Source: CAD feature listing. Evaluate the final solid. Frame: model axes, mm. A direction names the side the tool comes from. Coordinates: 2 decimals unless noted, no trailing zeros. Loops run counter-clockwise (first coordinate to the right, second up) from the corner with the lowest first, then second, coordinate; pieces in that order, holes last.
Solid Edge part; units mm, degrees
sketch "Sketch1" plane through (0, 0, 0) normal (0, 0, 1) x (1, 0, 0)
  line L0 (-500, -500) -> (500, -500)
  line L1 (500, -500) -> (500, 500)
  line L2 (500, 500) -> (-500, 500)
  line L3 (-500, 500) -> (-500, -500)
extrude "Protrusion1" add sketch "Sketch1" along normal blind 18
sketch "Sketch2" plane through (0, 0, 0) normal (0, 0, -1) x (1, 0, 0)
  circle A0 centre (0, 0) radius 450
extrude "Kihúzás_2" add sketch "Sketch2" along normal blind 18
sketch "Sketch3" plane through (0, 0, -18) normal (0, 0, -1) x (1, 0, 0)
  line L0 (-40.3424, -80.6848) -> (40.3424, -80.6848)
  line L1 (40.3424, -80.6848) -> (40.3424, 80.6848)
  line L2 (40.3424, 80.6848) -> (-40.3424, 80.6848)
  line L3 (-40.3424, 80.6848) -> (-40.3424, -80.6848)
extrude "Kihúzás_5" add sketch "Sketch3" along normal blind 5
sketch "Sketch4" plane through (0, 0, -23) normal (0, 0, -1) x (0, 1, 0)
  circle A0 centre (0, 0) radius 10
extrude "Kihúzás_6" add sketch "Sketch4" along normal blind 65
sketch "Sketch5" plane through (0, 0, 18) normal (0, 0, 1) x (0, -1, 0)
  line L0 (-500, -500) -> (500, -500)
  line L1 (500, -500) -> (500, 500)
  line L2 (500, 500) -> (-500, 500)
  line L3 (-500, 500) -> (-500, -500)
  line L4 (-518, -518) -> (518, -518)
  line L5 (518, -518) -> (518, 518)
  line L6 (518, 518) -> (-518, 518)
  line L7 (-518, 518) -> (-518, -518)
extrude "Kihúzás_9" add sketch "Sketch5" against normal blind 68
sketch "Sketch6" plane through (0, 0, 18) normal (0, 0, 1) x (0, -1, 0)
  line L0 (-500, -500) -> (500, -500)
  line L1 (500, -500) -> (500, 500)
  line L2 (500, 500) -> (-500, 500)
  line L3 (-500, 500) -> (-500, -500)
  line L4 (-518, -518) -> (518, -518)
  line L5 (518, -518) -> (518, 518)
  line L6 (518, 518) -> (-518, 518)
  line L7 (-518, 518) -> (-518, -518)
extrude "Kihúzás_10" add sketch "Sketch6" along normal blind 42
Q1. Section query B-B on x = 302. Return the cut outline in (y, z), then the cut area to 3 significant figures.
Q2. Section query A-A on z = 35. Return the cut outline in (x, y), then the cut area to 3 significant figures.
Q3. First-contact query: pin 1 Ø1.5 at (x, y) = (245, -223) entering from -Z. Flat tip, straight axial feed; report the tip coordinate or a pass-through.
Q4. Draft query along Y for faces 1 (the flat face through (-501, 233, 60)), 2 (the flat face through (7, 518, 6)), 3 (the flat face through (-7, 7, 18)). Return one class per face: released by +Y, released by -Y, zero draft, split by the parting line, or undercut.
Q5. Material intervals for line 1 along X through (y, z) = (-462, -29); line 2 along Z through (x, y) = (-212, -208), sorted ascending.
Q6. Reachability of faces 4 (the flat face through (500, -7, 39)), 5 (the flat face through (18, 1, -23)), 6 (the flat face through (-518, 7, 6)) from +Z, -Z, +X, -X, +Y, -Y: full face, straight path, thin tool, end or side. Return the list, or none.
Q7. Section query C-C on y = -277.5. Return the cut outline in (x, z).
Resolved:
1. outline: (-518, -50) - (-500, -50) - (-500, 0) - (-333.61, 0) - (-333.61, -18) - (333.61, -18) - (333.61, 0) - (500, 0) - (500, -50) - (518, -50) - (518, 60) - (500, 60) - (500, 18) - (-500, 18) - (-500, 60) - (-518, 60) - close
1. area: 34,000 mm2
2. outline: (-518, -518) - (518, -518) - (518, 518) - (-518, 518) - close; hole (-500, -500) - (500, -500) - (500, 500) - (-500, 500) - close
2. area: 73,300 mm2
3. pin 1: stops at z = -18
4. face 1: zero draft
4. face 2: released by +Y
4. face 3: undercut
5. line 1: x = -518 to -500, 500 to 518
5. line 2: z = -18 to 18
6. face 4: +Z
6. face 5: -Z
6. face 6: +Z, -Z, -X, +Y, -Y
7. outline: (-518, -50) - (-500, -50) - (-500, 0) - (-354.25, 0) - (-354.25, -18) - (354.25, -18) - (354.25, 0) - (500, 0) - (500, -50) - (518, -50) - (518, 60) - (500, 60) - (500, 18) - (-500, 18) - (-500, 60) - (-518, 60) - close
